CAD build for the part. Positions are in the model's coordinates, mm. Give positions to 0.01 mm unless a question says otherwise; leave off trailing zeros. Write each loop counter-clockwise with the first axis right and the second up, starting at its lowest first coordinate (ties: lowest second). Pieces come first, ordered by that corner, then holes. Notation, with made-up numbers: (44, 86.5) -> (95, 86.5) arc R32 ccw to (95, 121.5) -> close; hole circle Ø10 at (59.25, -14.75). An arc over 180 degrees is marked (long way). Use one line per item in the form item = value. Start each with the question number.
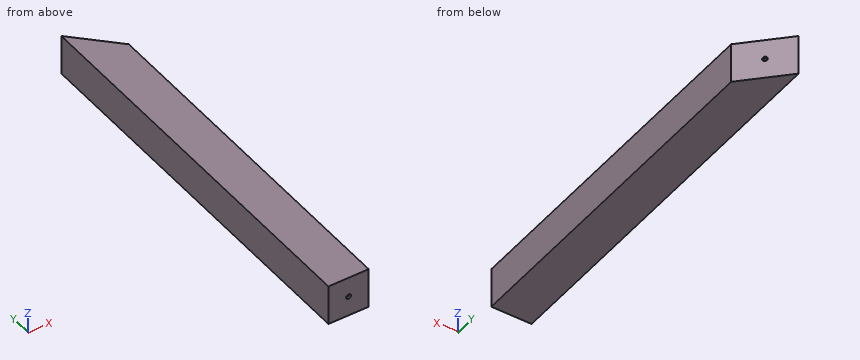
from build123d import *

# Parameters (mm, degrees)
SKETCH1_W                                         = 25.4
SKETCH1_H                                         = 25.4
BOSS_EXTRUDE1_DEPTH                               = 124.485
F_0_80_TAPPED_HOLE1_D                             = 1.19126
F_0_80_TAPPED_HOLE1_DEPTH                         = 20
F_0_80_TAPPED_HOLE1_CSINK_D                       = 3.0226
F_0_80_TAPPED_HOLE1_CSINK_ANGLE                   = 100
F_0_80_TAPPED_HOLE1_TIP                           = 0.357890611
CUT_EXTRUDE1_DEPTH                                = 13.7
CUT_EXTRUDE1_DEPTH_BACK                           = 13.7
CSK_FOR_0_FLAT_HEAD_MACHINE_SCREW_100_D           = 1.778
CSK_FOR_0_FLAT_HEAD_MACHINE_SCREW_100_DEPTH       = 10
CSK_FOR_0_FLAT_HEAD_MACHINE_SCREW_100_CSINK_D     = 3.0226
CSK_FOR_0_FLAT_HEAD_MACHINE_SCREW_100_CSINK_ANGLE = 100
CSK_FOR_0_FLAT_HEAD_MACHINE_SCREW_100_TIP         = 0.53416509


with BuildPart() as part:
    # Sketch1 → Boss-Extrude1 (new body, symmetric)
    with BuildSketch(Plane(origin=(0, 0, 0), x_dir=(1, 0, 0), z_dir=(0, 1, 0))):
        Rectangle(SKETCH1_W, SKETCH1_H)
    extrude(amount=BOSS_EXTRUDE1_DEPTH, both=True)

    # #0-80 Tapped Hole1
    with Locations(Plane(origin=(0, -124.485, 0), x_dir=(-1, 0, 0), z_dir=(0, -1, 0))):
        with Locations((0, 0)):
            CounterSinkHole(F_0_80_TAPPED_HOLE1_D / 2, F_0_80_TAPPED_HOLE1_CSINK_D / 2, depth=F_0_80_TAPPED_HOLE1_DEPTH, counter_sink_angle=F_0_80_TAPPED_HOLE1_CSINK_ANGLE)
            with Locations((0, 0, -(F_0_80_TAPPED_HOLE1_DEPTH + F_0_80_TAPPED_HOLE1_TIP / 2))):  # 118° drill point
                Cone(0, F_0_80_TAPPED_HOLE1_D / 2, F_0_80_TAPPED_HOLE1_TIP, mode=Mode.SUBTRACT)

    # Sketch4 → Cut-Extrude1 (cut, two sides)
    with BuildSketch(Plane.XY) as cut_extrude1_sk:
        Polygon((12.7, 124.485), (-12.7, 124.485), (12.7, 99.085), align=None)
    extrude(amount=CUT_EXTRUDE1_DEPTH, mode=Mode.SUBTRACT)
    extrude(cut_extrude1_sk.sketch, amount=-CUT_EXTRUDE1_DEPTH_BACK, mode=Mode.SUBTRACT)

    # CSK for #0 Flat Head Machine Screw (100)1
    with Locations(Plane(origin=(55.8925, 55.8925, 0), x_dir=(0.707106781, -0.707106781, 0), z_dir=(0.707106781, 0.707106781, 0))):
        with Locations((-79.043931535, 0)):
            CounterSinkHole(CSK_FOR_0_FLAT_HEAD_MACHINE_SCREW_100_D / 2, CSK_FOR_0_FLAT_HEAD_MACHINE_SCREW_100_CSINK_D / 2, depth=CSK_FOR_0_FLAT_HEAD_MACHINE_SCREW_100_DEPTH, counter_sink_angle=CSK_FOR_0_FLAT_HEAD_MACHINE_SCREW_100_CSINK_ANGLE)
            with Locations((0, 0, -(CSK_FOR_0_FLAT_HEAD_MACHINE_SCREW_100_DEPTH + CSK_FOR_0_FLAT_HEAD_MACHINE_SCREW_100_TIP / 2))):  # 118° drill point
                Cone(0, CSK_FOR_0_FLAT_HEAD_MACHINE_SCREW_100_D / 2, CSK_FOR_0_FLAT_HEAD_MACHINE_SCREW_100_TIP, mode=Mode.SUBTRACT)


solid = part.part
1) Wall check: line 1 along Z through (x, y) = (0, -113.75); line 2 along Y through (x, z) = (-6.75, -5) (3 decimals); line 3 along Y through (x, z) = (0, -8.75) (3 decimals). Give the ranges that are in metal, low to high. Write a range as from..to.
2) Cut at A-A (z = 8.25). Give the cut face in (x, y) (3 decimals), and give its area (3 significant figures).
3) Cut at B-B (x = 4.5). Give the cut face in (y, z) (3 decimals).
4) Pin check, flat tips, straight feed: pin 1 (12 mm diameter, centred on x = -2.5, z = 6, fed in from +Y) (3 decimals); pin 2 (1.4 mm diameter, centred on x = 0, z = 0, fed in from +Y); pin 3 (1 mm diameter, centred on x = -3, z = -8.5, fed in from +Y) (3 decimals). Stop position of each tip, or through.
Final values:
q1.line_1 = -12.7..-0.6, 0.6..12.7
q1.line_2 = -124.485..118.535
q1.line_3 = -124.485..111.785
q2.outline = (-12.7, -124.485) -> (12.7, -124.485) -> (12.7, 99.085) -> (-12.7, 124.485) -> close
q2.area = 6,000 mm^2
q3.outline = (-124.485, -12.7) -> (107.285, -12.7) -> (107.285, 12.7) -> (-124.485, 12.7) -> close
q4.pin_1 = 120.285
q4.pin_2 = 111.03
q4.pin_3 = 115.285
